The listing builds one solid part. Answer for the finished solid, in the listing's coordinates (mm). A direction names the side the tool comes from. Coordinates: 2 decimals unless noted, no trailing zeros. Write each loop counter-clockwise with the first axis right and the second up, starting at its lowest first coordinate (ties: lowest second). Pieces come first, ordered by that corner, then holes.
from build123d import *

# Parameters (mm, degrees)
F0_R      = 50.8
F1_DEPTH  = 203.2
F2_R      = 10.16
F1_FACE_R = 40.64
F3_DEPTH  = 48.514


with BuildPart() as f1:
    # F0 (on Top) → F1 (new body)
    with BuildSketch(Plane.XY):
        Circle(F0_R)
    extrude(amount=F1_DEPTH)

    # F2
    f2_edges = [f1.edges().sort_by_distance(p)[0] for p in [
        (-50.8, 0, 0),
        (50.8, 0, 101.6),
        (-50.8, 0, 203.2),
    ]]
    fillet(f2_edges, radius=F2_R)

    # F1_face (on face) → F3 (join)
    with BuildSketch(Plane.XY.offset(203.2)):
        Circle(F1_FACE_R)
    extrude(amount=F3_DEPTH)


solid = f1.part
1. A tool of negligible diameter and unlimited length cuts with its end or side. For faces 1 (the cylindrical face through (-11.012, -49.592, 100.32)), 2 (the cylindrical face through (-5.291, 40.294, 227.117)), from which of +Z, -Z, +X, -X, +Y, -Y can it reach the whole face along a straight path? Write none if from no direction.
Results found:
face 1: +Z, -Z
face 2: +Z
2. Section A-A on x = 0 is taken. Give the vertices of the cut face in (y, z).
Results found:
outline: (-50.8, 10.16) arc R10.16 ccw to (-40.64, 0) - (40.64, 0) arc R10.16 ccw to (50.8, 10.16) - (50.8, 193.04) arc R10.16 ccw to (40.64, 203.2) - (40.64, 251.71) - (-40.64, 251.71) - (-40.64, 203.2) arc R10.16 ccw to (-50.8, 193.04) - close
3. Section D-D on z = 195.5 is taken. Give the vertices of the cut face in (x, y), then the cut area to 3 significant figures.
Results found:
outline: circle Ø101 at (0, 0)
area: 8,010 mm2
4. Flat-ended cylindrical pins translate along their axes: P1, Ø12, axis at x = 38.5, z = 118.5, coming from the +Y side; P2, Ø10, axis at y = -10, z = 214, coming from the +X side; P3, Ø2, axis at x = 12, z = 122, coming from the +Y side. Find the tip coordinate at first contact, or state that the pin passes through.
Results found:
P1: stops at y = 39.04
P2: stops at x = 40.33
P3: stops at y = 49.59
5. Find the intervals of material crossed by L1, parallel to X at y = 1.5, z = 211.5; L2, parallel to Z at x = -20.5, y = -45; L3, parallel to X at y = -19.5, z = 183, in increasing order.
Results found:
L1: x = -40.61 to 40.61
L2: z = 5.1 to 198.1
L3: x = -46.91 to 46.91
6. Section C-C on z = 28.5 is taken. Give the vertices of the cut face in (x, y).
Results found:
outline: circle Ø101.6 at (0, 0)
